The listing builds one solid part. Answer for the finished solid, in the listing's coordinates (mm). Face numbers are marked on the shaded views. Round coordinates to 2 decimals unless told otherwise and drop trailing zeros. Order: outer loops, then holes, each group sorted by start corner. A loop starts at its lowest first (then second) coordinate and runs counter-clockwise, first axis right, second up. Notation, with made-up numbers: (-19, 87.5) - (-6, 87.5) arc R15 ccw to (-6, 91.5) - close; hole circle Ø2 at (80.5, 79.5). An arc over 180 degrees is marked (long way). Write item = value, one per line.
from build123d import *

# Parameters (mm, degrees)
TAP_DRILL_FOR_M3X0_5_TAP1_D = 2.5
CHAMFER1_SIZE               = 1
FILLET1_R                   = 0.5
FILLET2_R                   = 0.15


with BuildPart() as part:
    # Sketch1 → Revolve1 (revolve)
    with BuildSketch(Plane(origin=(0, 0, 0), x_dir=(1, 0, 0), z_dir=(0, 1, 0))):
        Polygon((0.79375, 0), (12, 0), (12, 4), (1.5875, 4), (1.5875, 8), (2, 8), (1.464101615, 10), (0.79375, 10), align=None)
    revolve(axis=Axis((0, 0, 0), (0, 0, -1)))

    # Tap Drill for M3x0.5 Tap1 (through all)
    with Locations(Plane.XY):
        with Locations((0, 8), (0, -8)):
            Hole(TAP_DRILL_FOR_M3X0_5_TAP1_D / 2)

    # Chamfer1
    chamfer1_edges = [part.edges().sort_by_distance(p)[0] for p in [
        (-12, 0, -4),
    ]]
    chamfer(chamfer1_edges, length=CHAMFER1_SIZE)

    # Fillet1
    fillet1_edges = [part.edges().sort_by_distance(p)[0] for p in [
        (-1.464101615, 0, -10),
        (-1.5875, 0, -4),
    ]]
    fillet(fillet1_edges, radius=FILLET1_R)

    # Fillet2
    fillet2_edges = [part.edges().sort_by_distance(p)[0] for p in [
        (-2, 0, -8),
        (-1.5875, 0, -8),
    ]]
    fillet(fillet2_edges, radius=FILLET2_R)


solid = part.part
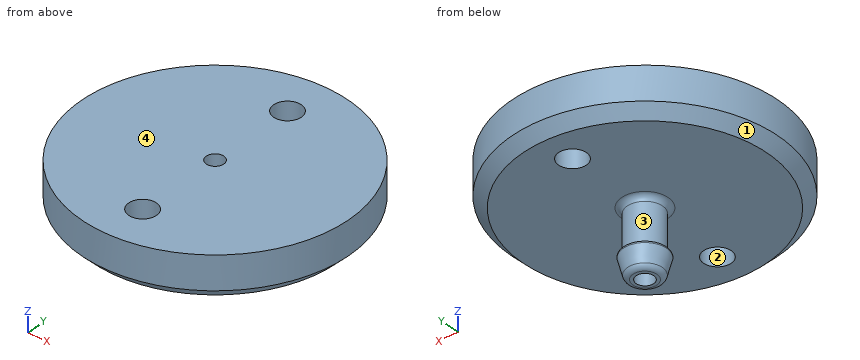
Q1. Section B-B on y = 0 is taken. Determine the outline of the cut face in (x, z), then the cut area to 3 significant figures.
Model answer:
outline = (-12, -3) - (-11, -4) - (-2.09, -4) arc R0.5 cw to (-1.59, -4.5) - (-1.59, -7.85) arc R0.15 cw to (-1.74, -8) - (-1.8, -8) arc R0.15 ccw to (-1.95, -8.19) - (-1.56, -9.63) arc R0.5 ccw to (-1.08, -10) - (-0.79, -10) - (-0.79, 0) - (-12, 0) - close; (0.79, -10) - (1.08, -10) arc R0.5 ccw to (1.56, -9.63) - (1.95, -8.19) arc R0.15 ccw to (1.8, -8) - (1.74, -8) arc R0.15 cw to (1.59, -7.85) - (1.59, -4.5) arc R0.5 cw to (2.09, -4) - (11, -4) - (12, -3) - (12, 0) - (0.79, 0) - close
area = 98.8 mm^2
Q2. Section C-C on z = -2.5 is taken. Determine the outline of the cut face in (x, y).
Model answer:
outline = circle Ø24 at (0, 0); hole circle Ø2.5 at (0, -8); hole circle Ø2.5 at (0, 8); hole circle Ø1.59 at (0, 0)
Q3. Find the intervals of material crossed by line 1 (Y direction, x = 0, z = -1); line 2 (Y direction, x = 0.25, z = -3.25); line 3 (X direction, y = 0, z = -7.75), in increasing order. Write a range as from..to.
Model answer:
line_1 = -12..-9.25, -6.75..-0.79, 0.79..6.75, 9.25..12
line_2 = -11.75..-9.22, -6.78..-0.75, 0.75..6.78, 9.22..11.75
line_3 = -1.59..-0.79, 0.79..1.59
Q4. Section D-D on z = -6 is taken. Determine the outline of the cut face in (x, y) (1 decimal).
Model answer:
outline = circle Ø3.2 at (0, 0); hole circle Ø1.6 at (0, 0)
Q5. Determine the mould class of the marked faces 1, 2, 3 and 4 for opening direction Z: released by +Z, released by -Z, zero draft, split by the parting line, or undercut.
Model answer:
face_1 = released by -Z
face_2 = zero draft
face_3 = undercut
face_4 = released by +Z
Q6. Flat-ended cylindrical pins translate along their axes: P1, Ø1, axis at y = 0.5, z = -7, coming from the +X side; P2, Ø1, axis at x = 0, y = 0, coming from the +Z side; P3, Ø1, axis at x = -3.5, y = 6, coming from the -Z side; P4, Ø2, axis at x = 4, z = -4.5, coming from the +Y side. Find the tip coordinate at first contact, or state that the pin passes through.
Model answer:
P1 = 1.59
P2 = through
P3 = -4
P4 = 10.84
Q7. Section A-A on x = 0 is taken. Count the separate pieces of the cut face and the enclosed holes in it, then the cut area to 3 significant figures.
Model answer:
separate_pieces = 4
enclosed_holes = 0
area = 78.8 mm^2
